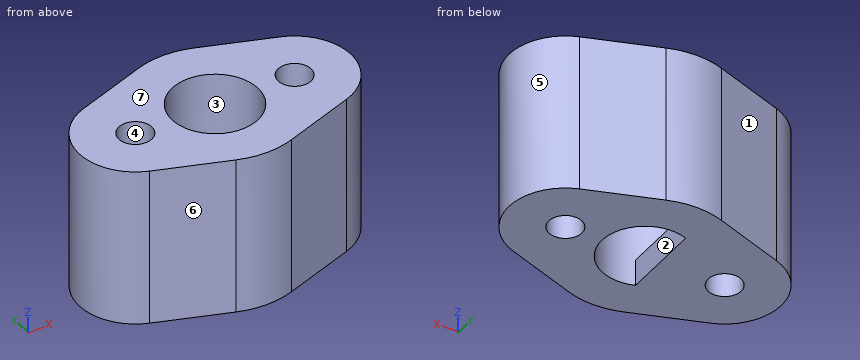
from build123d import *

# Parameters (mm, degrees)
F0_R     = 1.25
F0_R_2   = 3.25
F1_DEPTH = 12
F3_DEPTH = 2


with BuildPart() as f1:
    # F0 (on Top) → F1 (new body)
    with BuildSketch(Plane.XY):
        with BuildLine():
            ThreePointArc((7.416667, -4.006938), (10.25, 0), (7.416667, 4.006938))
            Line((7.416667, 4.006938), (2.083333, 5.892557))
            ThreePointArc((2.083333, 5.892557), (0, 6.25), (-2.083333, 5.892557))
            Line((-2.083333, 5.892557), (-7.416667, 4.006938))
            ThreePointArc((-7.416667, 4.006938), (-10.25, 0), (-7.416667, -4.006938))
            Line((-7.416667, -4.006938), (-2.083333, -5.892557))
            ThreePointArc((-2.083333, -5.892557), (0, -6.25), (2.083333, -5.892557))
            Line((2.083333, -5.892557), (7.416667, -4.006938))
        make_face()
        with Locations((-6, 0)):
            Circle(F0_R, mode=Mode.SUBTRACT)
        Circle(F0_R_2, mode=Mode.SUBTRACT)
        with Locations((6, 0)):
            Circle(F0_R, mode=Mode.SUBTRACT)
    extrude(amount=F1_DEPTH)

    # F2 (on face) → F3 (join)
    with BuildSketch(Plane(origin=(0, 0, 0), x_dir=(1, 0, 0), z_dir=(0, 0, -1))):
        with BuildLine():
            Line((-1.179652, -3.028353), (-1.179652, 3.028353))
            ThreePointArc((-1.179652, 3.028353), (-3.25, 0), (-1.179652, -3.028353))
        make_face()
    extrude(amount=-F3_DEPTH)


solid = f1.part
Check sheet for the modelled part. Datum: model origin and axes. Units: mm. Face numbers are marked on the shaded views. A direction names the side the tool comes from. Round coordinates to 2 decimals unless told otherwise and drop trailing zeros. Loops run counter-clockwise (first coordinate to the right, second up) from the corner with the lowest first, then second, coordinate; pieces in that order, holes last. Notation, with made-up numbers: (51.25, -38) -> (89.25, -38) arc R27 cw to (89.25, -19) -> close; hole circle Ø11 at (56.5, -18.75). An arc over 180 degrees is marked (long way). Put each result on its own line as item: value. Start each with the question number.
1. Access from +Z, -Z, +X, -X, +Y, -Y to the whole of each face (thin tool, end or side, straight path). Record for the marked faces 1, 2 and 3.
2. Draft check along X on the marked faces 4, 5, 6 and 7. Enter one of: +X half, -X half, draft (parallel to the pull), parting line (faces both ways), or undercut.
3. Section check A-A (y = 0). Enter the section's corners in (x, z), plus the area to 3 significant figures.
4. Section check C-C (z = 4.5). Enter the section's corners in (x, y), plus the area to 3 significant figures.
5. Scan lines: probe 1 along Y at (x, z) = (0, 8.5); probe 2 along X at (y, z) = (-0.5, 6.5); probe 3 along Y at (x, z) = (-5.5, 3.75). Record each from-to range of solid material in increasing order.
6. Section check D-D (z = 1.75). Enter the section's corners in (x, y), plus the area to 3 significant figures.
7. Gauge pin test, flat ends, axial feed: pin 1 (1 mm diameter, centred on x = 4.5, z = 8, fed in from -Y); pin 2 (1 mm diameter, centred on x = -0.5, y = -3, fed in from +Z); pin 3 (6 mm diameter, centred on x = 0, y = 0, fed in from +Z); pin 4 (3 mm diameter, centred on x = -7, z = 6.5, fed in from +Y). Record the tip position at first contact, or that the pin passes through.
8. Section check B-B (x = 0). Enter the section's corners in (y, z), plus the area to 3 significant figures.
Findings:
1. face 1: +Z, -Z, -X, +Y
1. face 2: +Z, -Z
1. face 3: +Z
2. face 4: undercut
2. face 5: +X half
2. face 6: -X half
2. face 7: draft
3. outline: (-10.25, 0) -> (-7.25, 0) -> (-7.25, 12) -> (-10.25, 12) -> close; (-4.75, 0) -> (-1.18, 0) -> (-1.18, 2) -> (-3.25, 2) -> (-3.25, 12) -> (-4.75, 12) -> close; (3.25, 0) -> (4.75, 0) -> (4.75, 12) -> (3.25, 12) -> close; (7.25, 0) -> (10.25, 0) -> (10.25, 12) -> (7.25, 12) -> close
3. area: 112 mm^2
4. outline: (-7.42, -4.01) -> (-2.08, -5.89) arc R6.25 ccw to (2.08, -5.89) -> (7.42, -4.01) arc R4.25 ccw to (7.42, 4.01) -> (2.08, 5.89) arc R6.25 ccw to (-2.08, 5.89) -> (-7.42, 4.01) arc R4.25 ccw to start; hole circle Ø2.5 at (-6, 0); hole circle Ø6.5 at (0, 0); hole circle Ø2.5 at (6, 0)
4. area: 147 mm^2
5. probe 1: y = -6.25 to -3.25, 3.25 to 6.25
5. probe 2: x = -10.22 to -7.15, -4.85 to -3.21, 3.21 to 4.85, 7.15 to 10.22
5. probe 3: y = -4.68 to -1.15, 1.15 to 4.68
6. outline: (-7.42, -4.01) -> (-2.08, -5.89) arc R6.25 ccw to (2.08, -5.89) -> (7.42, -4.01) arc R4.25 ccw to (7.42, 4.01) -> (2.08, 5.89) arc R6.25 ccw to (-2.08, 5.89) -> (-7.42, 4.01) arc R4.25 ccw to start; hole circle Ø2.5 at (-6, 0); hole (-1.18, -3.03) arc R3.25 ccw (long way) to (-1.18, 3.03) -> close; hole circle Ø2.5 at (6, 0)
6. area: 156 mm^2
7. pin 1: stops at y = -5.21
7. pin 2: stops at z = 12
7. pin 3: stops at z = 2
7. pin 4: stops at y = 4.68
8. outline: (-6.25, 0) -> (-3.25, 0) -> (-3.25, 12) -> (-6.25, 12) -> close; (3.25, 0) -> (6.25, 0) -> (6.25, 12) -> (3.25, 12) -> close
8. area: 72.0 mm^2
